Model file for the job. Use its own axes, mm. A direction names the side the tool comes from. Coordinates: 2 decimals unless noted, no trailing zeros. Loops run counter-clockwise (first coordinate to the right, second up) from the corner with the lowest first, then second, coordinate; pieces in that order, holes last.
from build123d import *

# Parameters (mm, degrees)
SKETCH1_W           = 26
SKETCH1_H           = 26
SKETCH1_R           = 1.15
SKETCH1_R_2         = 0.95
SKETCH1_W_2         = 12.1
SKETCH1_H_2         = 6.1
BOSS_EXTRUDE1_DEPTH = 4
SKETCH7_W           = 26
SKETCH7_H           = 26
SKETCH7_R           = 0.95
SKETCH7_R_2         = 1.15
BOSS_EXTRUDE4_DEPTH = 1
SKETCH8_R           = 2.1
CUT_EXTRUDE5_DEPTH  = 2.2
SKETCH3_W           = 5.4
SKETCH3_H           = 1.5
CUT_EXTRUDE6_DEPTH  = 4
CHAMFER2_SIZE       = 1.5
FILLET1_R           = 1


with BuildPart() as part:
    # Sketch1 → Boss-Extrude1 (new body)
    with BuildSketch(Plane.XY):
        with Locations((-1, 1)):
            Rectangle(SKETCH1_W, SKETCH1_H)
        with Locations((-11, 11)):
            Circle(SKETCH1_R, mode=Mode.SUBTRACT)
        with Locations((9, 11)):
            Circle(SKETCH1_R, mode=Mode.SUBTRACT)
        with Locations((9, -9)):
            Circle(SKETCH1_R, mode=Mode.SUBTRACT)
        with Locations((-11, -9)):
            Circle(SKETCH1_R, mode=Mode.SUBTRACT)
        with Locations((7.5, 6.5)):
            Circle(SKETCH1_R_2, mode=Mode.SUBTRACT)
        with Locations((-7.5, -6.5)):
            Circle(SKETCH1_R_2, mode=Mode.SUBTRACT)
        with Locations((0.55, -4.65)):
            Rectangle(SKETCH1_W_2, SKETCH1_H_2, mode=Mode.SUBTRACT)
    extrude(amount=BOSS_EXTRUDE1_DEPTH)

    # Sketch7 → Boss-Extrude4 (add)
    with BuildSketch(Plane.XY.offset(4)):
        with Locations((-1, 1)):
            Rectangle(SKETCH7_W, SKETCH7_H)
        with Locations((7.5, 6.5)):
            Circle(SKETCH7_R, mode=Mode.SUBTRACT)
        with Locations((-7.5, -6.5)):
            Circle(SKETCH7_R, mode=Mode.SUBTRACT)
        with Locations((-11, -9)):
            Circle(SKETCH7_R_2, mode=Mode.SUBTRACT)
        with Locations((9, -9)):
            Circle(SKETCH7_R_2, mode=Mode.SUBTRACT)
        with Locations((9, 11)):
            Circle(SKETCH7_R_2, mode=Mode.SUBTRACT)
        with Locations((-11, 11)):
            Circle(SKETCH7_R_2, mode=Mode.SUBTRACT)
    extrude(amount=BOSS_EXTRUDE4_DEPTH)

    # Sketch8 → Cut-Extrude5 (cut)
    with BuildSketch(Plane(origin=(0, 0, 0), x_dir=(-1, 0, 0), z_dir=(0, 0, -1))):
        with Locations((-9, 11)):
            Circle(SKETCH8_R)
        with Locations((11, 11)):
            Circle(SKETCH8_R)
        with Locations((11, -9)):
            Circle(SKETCH8_R)
        with Locations((-9, -9)):
            Circle(SKETCH8_R)
    extrude(amount=-CUT_EXTRUDE5_DEPTH, mode=Mode.SUBTRACT)

    # Sketch3 → Cut-Extrude6 (cut)
    with BuildSketch(Plane(origin=(0, 0, 0), x_dir=(-1, 0, 0), z_dir=(0, 0, -1))):
        with Locations((-9.3, -4.65)):
            Rectangle(SKETCH3_W, SKETCH3_H)
    extrude(amount=-CUT_EXTRUDE6_DEPTH, mode=Mode.SUBTRACT)

    # Chamfer2
    chamfer2_edges = [part.edges().sort_by_distance(p)[0] for p in [
        (6.6, -5.4, 2),
        (6.6, -3.9, 2),
    ]]
    chamfer(chamfer2_edges, length=CHAMFER2_SIZE)

    # Fillet1
    fillet1_edges = [part.edges().sort_by_distance(p)[0] for p in [
        (12, -12, 2.5),
        (-14, -12, 2.5),
        (-14, 14, 2.5),
        (12, 14, 2.5),
    ]]
    fillet(fillet1_edges, radius=FILLET1_R)


solid = part.part
Q1. Mould opens along X. For faces 1 (the cylindrical face through (-13.699, 13.715, 2.465)), 2 (the flat face through (10, -3.9, 2)), 3 (the flat face through (0, -7.7, 2)), 4 (the flat face through (7.3, -3.1, 2)) say: +X half, -X half, draft (parallel to the pull), parting line (faces both ways), or undercut.
Answers:
face 1: -X half
face 2: draft
face 3: undercut
face 4: undercut
Q2. Drill centre lines: line 1 (X direction, y = 11, z = 4.15); line 2 (Y direction, x = 10.5, z = 2.4); line 3 (Y direction, x = -9.25, z = 0.9). Where is each one in solid material? Low to high.
Answers:
line 1: x = -14 to -12.15, -9.85 to 7.85, 10.15 to 12
line 2: y = -12 to -5.4, -3.9 to 14
line 3: y = -12 to -10.16, -7.84 to 9.84, 12.16 to 14
Q3. Slice it at A-A (y = 6.5). List the corners of the cut face in (x, z).
Answers:
outline: (-14, 0) - (6.55, 0) - (6.55, 5) - (-14, 5) - close; (8.45, 0) - (12, 0) - (12, 5) - (8.45, 5) - close
Q4. Slice it at B-B (x = 9). List the corners of the cut face in (y, z), and give its area (3 significant figures).
Answers:
outline: (-12, 0) - (-11.1, 0) - (-11.1, 2.2) - (-10.15, 2.2) - (-10.15, 5) - (-12, 5) - close; (-7.85, 2.2) - (-6.9, 2.2) - (-6.9, 0) - (-5.4, 0) - (-5.4, 4) - (-3.9, 4) - (-3.9, 0) - (8.9, 0) - (8.9, 2.2) - (9.85, 2.2) - (9.85, 5) - (-7.85, 5) - close; (12.15, 2.2) - (13.1, 2.2) - (13.1, 0) - (14, 0) - (14, 5) - (12.15, 5) - close
area: 92.6 mm2
Q5. Which spindle directions (+Z, -Z, +X, -X, +Y, -Y) get a long thin tool onto all of the face, cutting with end or side? Do faces 5 (the flat face through (12, 1, 2)), 6 (the cylindrical face through (-8.9, 11.09, 1.08)), 7 (the flat face through (10, -5.4, 2)). Say none if no direction does.
Answers:
face 5: +Z, -Z, +X, +Y, -Y
face 6: -Z
face 7: -Z, +X
Q6. Slice it at C-C (y = -9). List the corners of the cut face in (x, z), and give its area (3 significant figures).
Answers:
outline: (-14, 0) - (-13.1, 0) - (-13.1, 2.2) - (-12.15, 2.2) - (-12.15, 5) - (-14, 5) - close; (-9.85, 2.2) - (-8.9, 2.2) - (-8.9, 0) - (6.9, 0) - (6.9, 2.2) - (7.85, 2.2) - (7.85, 5) - (-9.85, 5) - close; (10.15, 2.2) - (11.1, 2.2) - (11.1, 0) - (12, 0) - (12, 5) - (10.15, 5) - close
area: 98.6 mm2
Q7. Flat gauge pin, fed straight in: P1, Ø3, axis at x = -11, y = 11, coming from the -Z side. Where does the tip first touch, or does it go through?
Answers:
P1: stops at z = 2.2
Q8. Slice it at D-D (x = -7.5). List the corners of the cut face in (y, z), and give its area (4 significant figures).
Answers:
outline: (-12, 0) - (-7.45, 0) - (-7.45, 5) - (-12, 5) - close; (-5.55, 0) - (14, 0) - (14, 5) - (-5.55, 5) - close
area: 120.5 mm2
